Source: CAD feature listing. Evaluate the final solid. Frame: model axes, mm. Face numbers are marked on the shaded views. A direction names the side the tool comes from. Coordinates: 2 decimals unless noted, no trailing zeros. Loops run counter-clockwise (first coordinate to the right, second up) from the corner with the lowest first, then second, coordinate; pieces in that order, holes last. Notation, with made-up numbers: (61, -13.75) -> (66, -13.75) arc R12 cw to (66, 8.25) -> close; hole circle Ø3 at (76.5, 68). An arc over 180 degrees is marked (long way). Answer as CSV lines item,"result".
from build123d import *

# Parameters (mm, degrees)
F0_R     = 22.026537
F1_DEPTH = 84.582
F2_R     = 6.35
F3_DEPTH = 45.72
F4_R     = 21.464909
F5_DEPTH = 35.56
F6_R     = 2.691467
F6_R_2   = 2.446789
F6_W     = 16.638168
F6_H     = 8.80844
F7_DEPTH = 3.81


with BuildPart() as f1:
    # F0 (on Front) → F1 (new body)
    with BuildSketch(Plane.XZ):
        with Locations((0, 2.20211)):
            Circle(F0_R)
    extrude(amount=F1_DEPTH)

    # F2 (on Top) → F3 (join)
    with BuildSketch(Plane.XY):
        with Locations((-11.390769, -17.843104)):
            Circle(F2_R)
        with Locations((11.357995, -17.872222)):
            Circle(F2_R)
        with Locations((-10.32545, -68.983197)):
            Circle(F2_R)
        with Locations((11.616129, -68.725064)):
            Circle(F2_R)
    extrude(amount=F3_DEPTH)

    # F4 (on face) → F5 (join)
    with BuildSketch(Plane.XZ.offset(84.582)):
        with Locations((0, -7.095688)):
            Circle(F4_R)
    extrude(amount=F5_DEPTH)

    # F6 (on face) → F7 (cut)
    with BuildSketch(Plane.XZ.offset(120.142)):
        with Locations((-9.787156, -16.882844)):
            Circle(F6_R)
        with Locations((8.319084, -16.882844)):
            Circle(F6_R_2)
        Rectangle(F6_W, F6_H)
    extrude(amount=-F7_DEPTH, mode=Mode.SUBTRACT)


solid = f1.part
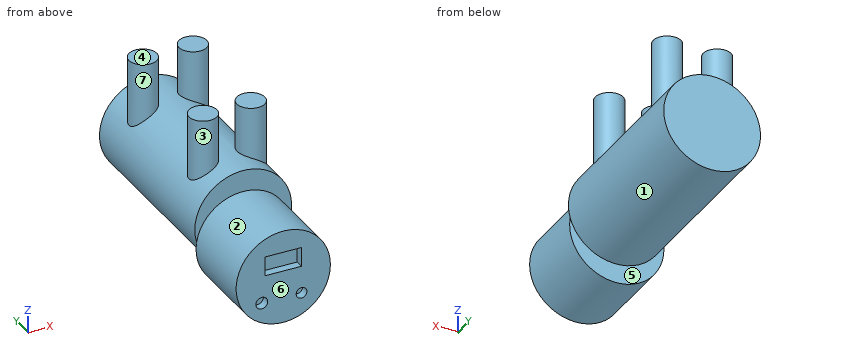
(1) Cut plane B-B (z = 11). Return the cut outline in (x, y).
Computed values:
outline,"(-20.19, -84.58) -> (-11.55, -84.58) -> (-11.55, -120.14) -> (11.55, -120.14) -> (11.55, -84.58) -> (20.19, -84.58) -> (20.19, 0) -> (-20.19, 0) -> close"
(2) Cut plane C-C (z = 39). Return the cut outline in (x, y), then the cut area to 3 significant figures.
Computed values:
outline,"circle Ø12.7 at (-11.39, -17.84); circle Ø12.7 at (-10.33, -68.98); circle Ø12.7 at (11.36, -17.87); circle Ø12.7 at (11.62, -68.73)"
area,"507 mm^2"
(3) Material intervals for L1, parallel to Y at x = -12.5, z = -24.5; L2, parallel to Y at x = 19.5, z = 4.5; L3, parallel to X at y = -19, z = 33, sorted ascending. Write a range as [from, to].
Computed values:
L1,"[-120.14, -84.58]"
L2,"[-84.58, 0]"
L3,"[-17.63, -5.15], [5.11, 17.61]"
(4) Cut plane A-A (x = 0). Return the cut outline in (y, z), then the cut area to 3 significant figures.
Computed values:
outline,"(-120.14, -28.56) -> (-84.58, -28.56) -> (-84.58, -19.82) -> (0, -19.82) -> (0, 24.23) -> (-84.58, 24.23) -> (-84.58, 14.37) -> (-120.14, 14.37) -> (-120.14, 4.4) -> (-116.33, 4.4) -> (-116.33, -4.4) -> (-120.14, -4.4) -> close"
area,"5,220 mm^2"
(5) Cut plane D-D (x = 12). Return the cut outline in (y, z).
Computed values:
outline,"(-120.14, -24.89) -> (-84.58, -24.89) -> (-84.58, -16.27) -> (0, -16.27) -> (0, 20.67) -> (-11.55, 20.67) -> (-11.55, 45.72) -> (-24.19, 45.72) -> (-24.19, 20.67) -> (-62.39, 20.67) -> (-62.39, 45.72) -> (-75.06, 45.72) -> (-75.06, 20.67) -> (-84.58, 20.67) -> (-84.58, 10.7) -> (-120.14, 10.7) -> close"
(6) Draft query along Y for the marked faces 4, 5, 6 and 7. Return one class per face: released by +Y, released by -Y, zero draft, split by the parting line, or undercut.
Computed values:
face 4,"zero draft"
face 5,"released by +Y"
face 6,"released by -Y"
face 7,"undercut"
(7) Pin query (flat end, axial travel): pin 1 Ø1 at (x, y) = (-4, -45) entering from -Z; pin 2 Ø1.5 at (x, z) = (7, -17) entering from -Y; pin 3 Ø5 at (y, z) = (-53, 15) entering from +X. Return the tip coordinate at first contact, or that it passes through.
Computed values:
pin 1,"z = -19.54"
pin 2,"y = -116.33"
pin 3,"x = 19.47"
(8) Access query for the marked faces 1, 2 and 3. Directions: +Z, -Z, +X, -X, +Y, -Y. A direction counts if a zero-diameter tool reaches every point of the face in a straight line with its end or side. Return the directions, or none.
Computed values:
face 1,"none"
face 2,"-Y"
face 3,"+Z"
